Check sheet for the drawn part. Datum: minimum x, y, z corner. Units: mm. Round coordinates to 2 decimals unless told otherwise and drop trailing zeros. Order: outer loops, then holes, each group sorted by start corner. A loop starts at its lowest first (then second) coordinate and runs counter-clockwise, first axis right, second up. Notation, with made-up numbers: (48.5, 68.25) -> (82.5, 68.25) arc R31 ccw to (82.5, 103.25) -> close; hole circle Ø8 at (-31.5, -4.75). An arc over 180 degrees is marked (long way). Answer in a Markdown table with one row per item.
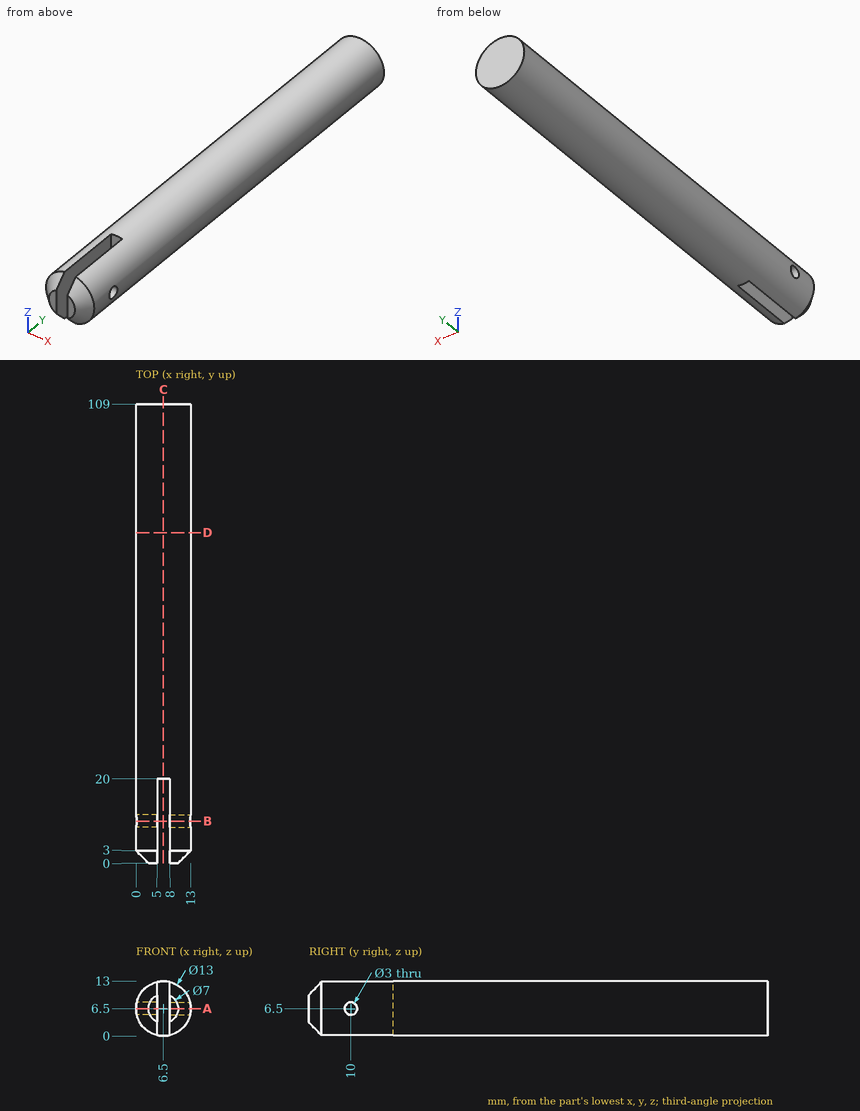
(1) Section check C-C on x = 6.5. Record the boundary of the cut face in (y, z).
Solutions:
| item | result |
|---|---|
| outline | (20, 0) -> (109, 0) -> (109, 13) -> (20, 13) -> close |
(2) Section check B-B on y = 10. Record the boundary of the cut face in (x, z).
Solutions:
| item | result |
|---|---|
| outline | (0.18, 5) arc R6.5 ccw to (5, 0.18) -> (5, 5) -> close; (0.18, 8) -> (5, 8) -> (5, 12.82) arc R6.5 ccw to start; (8, 0.18) arc R6.5 ccw to (12.82, 5) -> (8, 5) -> close; (8, 8) -> (12.82, 8) arc R6.5 ccw to (8, 12.82) -> close |
(3) Section check D-D on y = 78.5. Record the boundary of the cut face in (x, z), plus the area to 3 significant figures.
Solutions:
| item | result |
|---|---|
| outline | circle Ø13 at (6.5, 6.5) |
| area | 133 mm^2 |
(4) Section check A-A on z = 6.5. Record the boundary of the cut face in (x, y), plus the area to 3 significant figures.
Solutions:
| item | result |
|---|---|
| outline | (0, 3) -> (3, 0) -> (5, 0) -> (5, 8.5) -> (0, 8.5) -> close; (0, 11.5) -> (5, 11.5) -> (5, 20) -> (8, 20) -> (8, 11.5) -> (13, 11.5) -> (13, 109) -> (0, 109) -> close; (8, 0) -> (10, 0) -> (13, 3) -> (13, 8.5) -> (8, 8.5) -> close |
| area | 1,320 mm^2 |
(5) Depth check by flat-ended pin: pin 1 Ø4 at (x, z) = (10, 8.5) entering from -Y; pin 2 Ø3 at (x, y) = (6, 16) entering from +Z; pin 3 Ø5 at (y, z) = (68, 3) entering from +X; pin 4 Ø2 at (y, z) = (30.5, 4.5) entering from -X. Enter the tip coordinate at first touch or a pass-through.
Solutions:
| item | result |
|---|---|
| pin 1 | y = 0 |
| pin 2 | z = 12.82 |
| pin 3 | x = 12.92 |
| pin 4 | x = 0.08 |
(6) Scan lines: probe 1 along X at (y, z) = (7, 5); probe 2 along Y at (x, z) = (9.1, 6.5); probe 3 along Y at (x, z) = (5.25, 9.75). Record each from-to range of solid material in increasing order. Write a range as from..to.
Solutions:
| item | result |
|---|---|
| probe 1 | 0.18..5, 8..12.82 |
| probe 2 | 0..8.5, 11.5..109 |
| probe 3 | 20..109 |
